Geometry: final body of the model. Coordinates: model frame, mm. A direction names the side the tool comes from. Give positions to 0.01 mm unless a question says otherwise; leave off trailing zeros. Order: outer loops, then holes, each group sorted by start corner. A loop starts at its lowest first (then second) coordinate and runs counter-clockwise, first axis right, second up. Notation, with made-up numbers: (29, 32) - (81, 32) arc R18 cw to (81, 57) - close; hole circle Ø3 at (-13.5, 38.5). An arc over 180 degrees is marked (long way). Use one line per item in the form item = value.
from build123d import *

# Parameters (mm, degrees)
CROQUIS1_R              = 27.5
SALIENTE_EXTRUIR1_DEPTH = 10
CROQUIS4_R              = 4.05
CORTAR_EXTRUIR2_DEPTH   = 108
CROQUIS5_R              = 8.675
SALIENTE_EXTRUIR2_DEPTH = 5
CROQUIS6_R              = 4.05
CORTAR_EXTRUIR3_DEPTH   = 122


with BuildPart() as part:
    # Croquis1 → Saliente-Extruir1 (new, symmetric)
    with BuildSketch(Plane.XY):
        Circle(CROQUIS1_R)
    extrude(amount=SALIENTE_EXTRUIR1_DEPTH, both=True)

    # Croquis4 → Cortar-Extruir2 (cut)
    with BuildSketch(Plane.XY.offset(10)):
        Circle(CROQUIS4_R)
    extrude(amount=-CORTAR_EXTRUIR2_DEPTH, mode=Mode.SUBTRACT)

    # Croquis5 → Saliente-Extruir2 (add)
    with BuildSketch(Plane.XY.offset(10)):
        Circle(CROQUIS5_R)
    extrude(amount=SALIENTE_EXTRUIR2_DEPTH)

    # Croquis6 → Cortar-Extruir3 (cut, symmetric)
    with BuildSketch(Plane.XY.offset(15)):
        Circle(CROQUIS6_R)
    extrude(amount=CORTAR_EXTRUIR3_DEPTH, both=True, mode=Mode.SUBTRACT)


solid = part.part
(1) Reachability of faces 4 (the face through (-6.5, 6.5, 10)), 5 (the face through (4, -2, 15)) from +Z, -Z, +X, -X, +Y, -Y: full face, straight path, thin tool, end or side. Return the list, or none.
Computed values:
face_4 = +Z
face_5 = +Z, +X, -X, +Y, -Y
(2) Cut plane C-C on z = -4. Output: boundary loops of the cut face in (x, y).
Computed values:
outline = circle Ø55 at (0, 0); hole circle Ø8.1 at (0, 0)
(3) Ray query, line 1 along Y through (x, z) = (0, 9); line 2 along Z through (x, y) = (-6, -23); line 3 along Y through (x, z) = (-3.5, 2.5). Return the intervals inside material, ascending.
Computed values:
line_1 = -27.5 to -4.05, 4.05 to 27.5
line_2 = -10 to 10
line_3 = -27.28 to -2.04, 2.04 to 27.28
(4) Pull-direction query (Y, two-part tool) for faces 1 (the face through (-1.13, 8.6, 12.46)), 2 (the face through (-0.878, -3.954, 2.675)), 3 (the face through (0, -6, -10)); classes: released by +Y, released by -Y, zero draft, split by the parting line, or undercut.
Computed values:
face_1 = split by the parting line
face_2 = undercut
face_3 = zero draft
(5) Cut plane A-A on y = 0. Output: boundary loops of the cut face in (x, z) (3 decimals).
Computed values:
outline = (-27.5, -10) - (-4.05, -10) - (-4.05, 15) - (-8.675, 15) - (-8.675, 10) - (-27.5, 10) - close; (4.05, -10) - (27.5, -10) - (27.5, 10) - (8.675, 10) - (8.675, 15) - (4.05, 15) - close
(6) Cut plane D-D on y = -7. Output: boundary loops of the cut face in (x, z).
Computed values:
outline = (-26.59, -10) - (26.59, -10) - (26.59, 10) - (5.12, 10) - (5.12, 15) - (-5.12, 15) - (-5.12, 10) - (-26.59, 10) - close
(7) Contact query for flat-ended pins moving along their axis: pin 1 Ø1 at (x, z) = (22, -0.5) entering from -Y; pin 2 Ø12 at (x, z) = (-3.5, 5) entering from +Y; pin 3 Ø1 at (y, z) = (13, -4) entering from +X; pin 4 Ø7.5 at (x, y) = (0, 0) entering from +Z. Output: stop coordinate, or through.
Computed values:
pin_1 = -17.15
pin_2 = 27.5
pin_3 = 24.49
pin_4 = through
